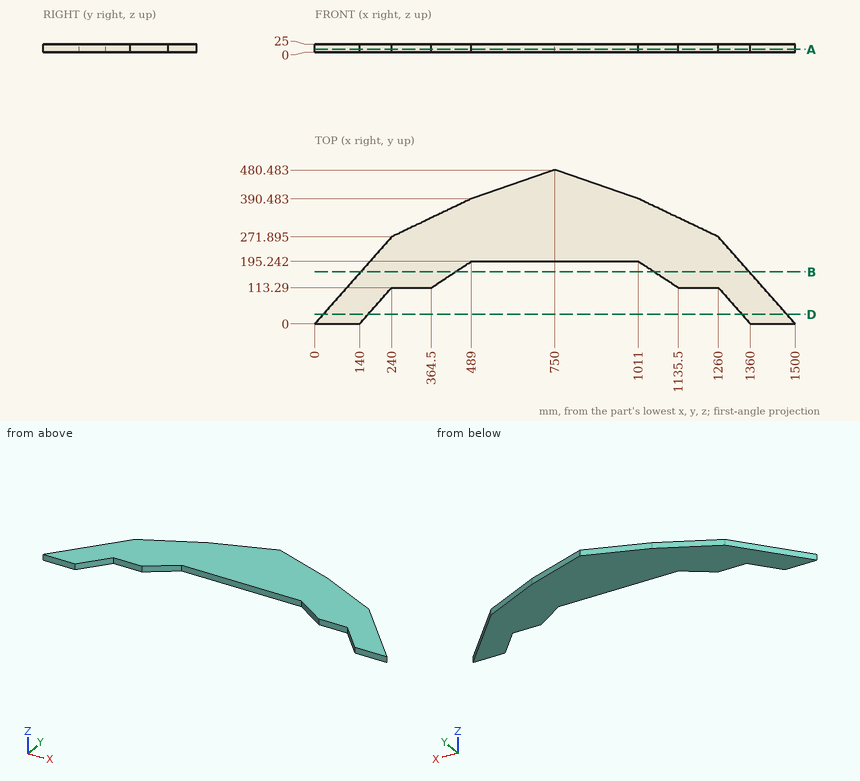
Verification items for this drawing (mm, ordinates from the low corner). Coordinates: 2 decimals unless noted, no trailing zeros. Order: outer loops, then holes, each group sorted by start corner. A loop starts at its lowest first (then second) coordinate and runs counter-clockwise, first axis right, second up.
Q1. Sectioned sample at A-A on z = 8.25. Record the cut outline in (x, y) (1 decimal).
Reply:
outline: (0, 0) - (140, 0) - (240, 113.3) - (364.5, 113.3) - (489, 195.2) - (1011, 195.2) - (1135.5, 113.3) - (1260, 113.3) - (1360, 0) - (1500, 0) - (1260, 271.9) - (1011, 390.5) - (750, 480.5) - (489, 390.5) - (240, 271.9) - close
Q2. Sectioned sample at D-D on y = 29.5. Record the cut outline in (x, z), and give its area (3 significant figures).
Reply:
outline: (26.04, 0) - (166.04, 0) - (166.04, 25) - (26.04, 25) - close; (1333.96, 0) - (1473.96, 0) - (1473.96, 25) - (1333.96, 25) - close
area: 7,000 mm2
Q3. Thickness scan on probe 1 along X at (y, z) = (142, 17.5) (1 decimal); probe 2 along X at (y, z) = (93, 10.75); probe 3 along Y at (x, z) = (468, 2.5). Record the ranges inside material, lowest first.
Reply:
probe 1: x = 125.3 to 408.1, 1091.9 to 1374.7
probe 2: x = 82.09 to 222.09, 1277.91 to 1417.91
probe 3: y = 181.42 to 380.48
Q4. Sectioned sample at B-B on y = 162. Record the cut outline in (x, z), and give its area (3 significant figures).
Reply:
outline: (143, 0) - (438.5, 0) - (438.5, 25) - (143, 25) - close; (1061.5, 0) - (1357, 0) - (1357, 25) - (1061.5, 25) - close
area: 14,800 mm2
Q5. Depth check by flat-ended pin: pin 1 Ø12.5 at (x, z) = (1222.5, 15.5) entering from -Y; pin 2 Ø2 at (y, z) = (232.5, 4.5) entering from -X (1 decimal); pin 3 Ø12 at (y, z) = (331, 11.5) entering from -X (1 decimal); pin 4 Ø1.5 at (x, y) = (1126, 180.5) entering from -Z. Enter the tip coordinate at first touch or a pass-through.
Reply:
pin 1: stops at y = 113.29
pin 2: stops at x = 204.3
pin 3: stops at x = 351.5
pin 4: stops at z = 0
